from build123d import *

# Parameters (mm, degrees)
BOSS_EXTRUDE1_DEPTH             = 33.909
CUT_EXTRUDE1_DEPTH              = 70.971972376
BOSS_EXTRUDE2_REACH             = 67.168
BOSS_EXTRUDE2_DIRECTION_2_REACH = 67.168
SKETCH3_R                       = 2.25
CUT_EXTRUDE2_DEPTH              = 62.483683724
SKETCH5_R                       = 4.125
CUT_EXTRUDE3_DEPTH              = 62.483683724
BOSS_EXTRUDE3_DEPTH             = 3.175
CHAMFER1_SIZE                   = 3.175
CUT_EXTRUDE4_DEPTH              = 81.960563335
CUT_EXTRUDE5_DEPTH              = 66.16805579
CUT_EXTRUDE5_DEPTH_BACK         = 66.16805579
SKETCH8_R                       = 2.54
SKETCH8_R_2                     = 1.7
SKETCH8_3_R                     = 11.0998
SKETCH8_3_R_2                   = 2.54
CUT_EXTRUDE6_DEPTH              = 2.286
CUT_EXTRUDE7_DEPTH              = 81.960563335
CUT_EXTRUDE7_DEPTH_BACK         = 81.960563335
SKETCH9_R                       = 4.445
SKETCH10_W                      = 15.875
SKETCH10_H                      = 11.092
BOSS_EXTRUDE4_DEPTH             = 8
CUT_EXTRUDE8_DEPTH              = 8
SKETCH12_W                      = 12.7
SKETCH12_H                      = 7.917
CUT_EXTRUDE9_DEPTH              = 18.286
CUT_EXTRUDE10_DEPTH             = 8
FILLET1_R                       = 0.79375
CUT_EXTRUDE11_REACH             = 71.954
CUT_EXTRUDE11_END_RADIUS        = 8.60425
SKETCH15_R                      = 1.5
CUT_EXTRUDE12_REACH             = 68.541
BOSS_EXTRUDE6_REACH             = 76.111


# Read off the part's stored shape, not the designer's step: Mirror1
with BuildPart() as part:
    # Sketch1 → Boss-Extrude1 (new, symmetric)
    with BuildSketch(Plane(origin=(0, 0, 0), x_dir=(0, 0, -1), z_dir=(1, 0, 0))):
        Polygon((0, -21.4015), (0, 19.8735), (4.7625, 19.8735), (4.7625, 11.8735), (51.3715, 11.8735), (51.3715, 0), (4.7625, 0), (4.7625, -21.4015), align=None)
    extrude(amount=BOSS_EXTRUDE1_DEPTH, both=True)

    # Sketch2 → Cut-Extrude1 (cut, symmetric)
    with BuildSketch(Plane(origin=(0, 11.8735, 0), x_dir=(1, 0, 0), z_dir=(0, 1, 0))):
        Polygon((33.909, 4.7625), (29.6545, 4.7625), (24.892, 9.525), (24.892, 42.644487102), (16.164987102, 51.3715), (23.7109, 51.3715), (33.909, 51.3715), align=None)
    extrude(amount=CUT_EXTRUDE1_DEPTH, both=True, mode=Mode.SUBTRACT)

    # Boss-Extrude2: up to this face of the body (flat: up to its plane)
    boss_extrude2_end = Plane(part.part.faces().sort_by_distance((0, -21.4015, -2.38125))[0])
    # Sketch4 → Boss-Extrude2 (add, up to the picked face)
    with BuildSketch(Plane.XZ, mode=Mode.PRIVATE) as boss_extrude2_sk1:
        Polygon((24.892, -9.525), (29.6545, -4.7625), (24.892, -4.7625), align=None)
    boss_extrude2_tool1 = split(extrude(boss_extrude2_sk1.sketch, amount=BOSS_EXTRUDE2_REACH, mode=Mode.PRIVATE), bisect_by=boss_extrude2_end, keep=Keep.BOTH, mode=Mode.PRIVATE)
    add(boss_extrude2_tool1.solids().sort_by(Axis((26.4795, 0, -6.35), (0, -1, 0)))[0])

    # Boss-Extrude2 direction 2: up to this face of the body (flat: up to its plane)
    boss_extrude2_direction_2_end = Plane(part.part.faces().sort_by_distance((0, 19.8735, -2.38125))[0])
    # Sketch4 → Boss-Extrude2 direction 2 (add, up to the picked face)
    with BuildSketch(Plane.XZ, mode=Mode.PRIVATE) as boss_extrude2_direction_2_sk1:
        Polygon((24.892, -9.525), (29.6545, -4.7625), (24.892, -4.7625), align=None)
    boss_extrude2_direction_2_tool1 = split(extrude(boss_extrude2_direction_2_sk1.sketch, amount=-BOSS_EXTRUDE2_DIRECTION_2_REACH, mode=Mode.PRIVATE), bisect_by=boss_extrude2_direction_2_end, keep=Keep.BOTH, mode=Mode.PRIVATE)
    add(boss_extrude2_direction_2_tool1.solids().sort_by(Axis((26.4795, 0, -6.35), (0, 1, 0)))[0])

    # Sketch3 → Cut-Extrude2 (cut, symmetric)
    with BuildSketch(Plane(origin=(0, 0, -4.7625), x_dir=(-1, 0, 0), z_dir=(0, 0, -1))):
        with Locations(Location((-29.4005, 10.3485, 0), (0, 0, 90))):
            Circle(SKETCH3_R)
        with Locations(Location((-29.4005, -11.8765, 0), (0, 0, 90))):
            Circle(SKETCH3_R)
        Polygon((-29.6545, 19.8735), (-33.909, 15.619), (-33.909, 19.8735), align=None)
        Polygon((-33.909, 5.078), (-29.6545, 0.8235), (-29.6545, -2.3515), (-33.909, -6.606), align=None)
        Polygon((-33.909, -17.147), (-29.6545, -21.4015), (-33.909, -21.4015), align=None)
    extrude(amount=CUT_EXTRUDE2_DEPTH, both=True, mode=Mode.SUBTRACT)

    # Sketch5 → Cut-Extrude3 (cut, through all)
    with BuildSketch(Plane(origin=(0, 0, -4.7625), x_dir=(-1, 0, 0), z_dir=(0, 0, -1))):
        with Locations((-29.4005, 10.3485)):
            Circle(SKETCH5_R)
        with Locations((-29.4005, -11.8765)):
            Circle(SKETCH5_R)
    extrude(amount=CUT_EXTRUDE3_DEPTH, mode=Mode.SUBTRACT)

    # Sketch6 → Boss-Extrude3 (add)
    with BuildSketch(Plane.ZY.offset(-24.892)):
        Polygon((-4.7625, -21.4015), (-4.7625, 0), (-42.644487102, 0), align=None)
    extrude(amount=BOSS_EXTRUDE3_DEPTH)

    # Chamfer1
    chamfer1_edges = [part.edges().sort_by_distance(p)[0] for p in [
        (21.717, -10.70075, -4.7625),
    ]]
    chamfer(chamfer1_edges, length=CHAMFER1_SIZE)

    # Sketch7 → Cut-Extrude4 (cut, symmetric)
    with BuildSketch(Plane(origin=(24.892, 0, 0), x_dir=(0, 0, -1), z_dir=(1, 0, 0))):
        Polygon((9.525, -18.71091665), (4.7625, -21.4015), (9.525, -21.4015), align=None)
    extrude(amount=CUT_EXTRUDE4_DEPTH, both=True, mode=Mode.SUBTRACT)

    # Mirror1
    split(bisect_by=Plane(origin=(0, 0, 0), x_dir=(0, 0, 1), z_dir=(1, 0, 0)), keep=Keep.TOP)

    # Mirror1 2: part across plane


with BuildPart() as part_1:
    add(part.part)
    add(part.part.mirror(Plane(origin=(0, 0, 0), x_dir=(0, 0, 1), z_dir=(1, 0, 0))))

    # Sketch8 → Cut-Extrude5 (cut, two sides: drawn at the far end of the back side and taken through both)
    with BuildSketch(Plane.XZ.offset(-CUT_EXTRUDE5_DEPTH_BACK)):
        with Locations(Location((0, -26.4795, 0), (0, 0, 270))):
            Circle(SKETCH8_R)
        with Locations(Location((15.5, -10.9795, 0), (0, 0, 270))):
            Circle(SKETCH8_R_2)
        with Locations(Location((15.5, -41.9795, 0), (0, 0, 270))):
            Circle(SKETCH8_R_2)
        with Locations(Location((-15.5, -41.9795, 0), (0, 0, 270))):
            Circle(SKETCH8_R_2)
        with Locations(Location((-15.5, -10.9795, 0), (0, 0, 270))):
            Circle(SKETCH8_R_2)
    extrude(amount=CUT_EXTRUDE5_DEPTH + CUT_EXTRUDE5_DEPTH_BACK, mode=Mode.SUBTRACT)

    # Sketch8<3> → Cut-Extrude6 (cut)
    with BuildSketch(Plane.XZ):
        with Locations(Location((0, -26.4795, 0), (0, 0, 270))):
            Circle(SKETCH8_3_R)
        with Locations(Location((0, -26.4795, 0), (0, 0, 270))):
            Circle(SKETCH8_3_R_2, mode=Mode.SUBTRACT)
    extrude(amount=-CUT_EXTRUDE6_DEPTH, mode=Mode.SUBTRACT)

    # Sketch9 → Cut-Extrude7 (cut, two sides: drawn at the far end of the back side and taken through both)
    with BuildSketch(Plane(origin=(24.892, 0, 0), x_dir=(0, 0, -1), z_dir=(1, 0, 0)).offset(-CUT_EXTRUDE7_DEPTH_BACK)):
        with Locations((35.8345, 11.8735)):
            Circle(SKETCH9_R)
    extrude(amount=CUT_EXTRUDE7_DEPTH + CUT_EXTRUDE7_DEPTH_BACK, mode=Mode.SUBTRACT)

    # Sketch10 → Boss-Extrude4 (add)
    with BuildSketch(Plane(origin=(0, 11.8735, 0), x_dir=(1, 0, 0), z_dir=(0, 1, 0))):
        with Locations((0, 45.8255)):
            Rectangle(SKETCH10_W, SKETCH10_H)
    extrude(amount=BOSS_EXTRUDE4_DEPTH)

    # Sketch11 → Cut-Extrude8 (cut)
    with BuildSketch(Plane(origin=(0, 11.8735, 0), x_dir=(1, 0, 0), z_dir=(0, 1, 0))):
        with BuildLine():
            Line((-7.9375, 40.2795), (7.9375, 40.2795))
            Line((7.9375, 40.2795), (11.26, 31.3895))
            Line((11.26, 31.3895), (11.26, 23.880766055))
            Line((11.26, 23.880766055), (2.086105319, 20.616574655))
            ThreePointArc((2.086105319, 20.616574655), (1.0584764, 20.347179337), (0, 20.2565))
            Line((0, 20.2565), (0, 17.87525))
            ThreePointArc((0, 17.87525), (-6.847467237, 21.26938383), (-8.292669268, 28.774005279))
            ThreePointArc((-8.292669268, 28.774005279), (-8.02669792, 30.069750228), (-7.9375, 31.3895))
            Line((-7.9375, 31.3895), (-7.9375, 40.2795))
        make_face()
    extrude(amount=-CUT_EXTRUDE8_DEPTH, mode=Mode.SUBTRACT)

    # Sketch12 → Cut-Extrude9 (cut)
    with BuildSketch(Plane.XZ):
        with Locations((0, -45.8255)):
            Rectangle(SKETCH12_W, SKETCH12_H)
    extrude(amount=-CUT_EXTRUDE9_DEPTH, mode=Mode.SUBTRACT)

    # Sketch13 → Cut-Extrude10 (cut)
    with BuildSketch(Plane(origin=(0, 11.8735, 0), x_dir=(1, 0, 0), z_dir=(0, 1, 0))):
        with BuildLine():
            Line((14.308, 21.730089687), (3.048, 17.723634801))
            Line((3.048, 17.723634801), (3.048, 15.232961596))
            ThreePointArc((3.048, 15.232961596), (-7.751371841, 17.779433066), (-11.522356749, 28.2145))
            Line((-11.522356749, 28.2145), (-21.717, 28.2145))
            Line((-21.717, 28.2145), (-21.717, 9.525))
            Line((-21.717, 9.525), (-21.717, 7.9375))
            Line((-21.717, 7.9375), (-20.152961933, 7.9375))
            ThreePointArc((-20.152961933, 7.9375), (-18.873886587, 8.584722111), (-18.637766637, 9.998644872))
            ThreePointArc((-18.637766637, 9.998644872), (-15.996109076, 14.229351079), (-12.2125, 10.9795))
            ThreePointArc((-12.2125, 10.9795), (-12.250148921, 10.483390924), (-12.362233363, 9.998644872))
            ThreePointArc((-12.362233363, 9.998644872), (-12.126113413, 8.584722111), (-10.847038067, 7.9375))
            Line((-10.847038067, 7.9375), (10.847038067, 7.9375))
            ThreePointArc((10.847038067, 7.9375), (12.126113413, 8.584722111), (12.362233363, 9.998644872))
            ThreePointArc((12.362233363, 9.998644872), (15.003890924, 14.229351079), (18.7875, 10.9795))
            ThreePointArc((18.7875, 10.9795), (18.749851079, 10.483390924), (18.637766637, 9.998644872))
            ThreePointArc((18.637766637, 9.998644872), (18.873886587, 8.584722111), (20.152961933, 7.9375))
            Line((20.152961933, 7.9375), (21.717, 7.9375))
            Line((21.717, 7.9375), (21.717, 9.525))
            Line((21.717, 9.525), (21.717, 28.2145))
            Line((21.717, 28.2145), (14.308, 28.2145))
            Line((14.308, 28.2145), (14.308, 21.730089687))
        make_face()
    extrude(amount=-CUT_EXTRUDE10_DEPTH, mode=Mode.SUBTRACT)

    # Fillet1
    fillet1_edges = [part_1.edges().sort_by_distance(p)[0] for p in [
        (3.048, 3.8735, -16.478298199),
        (8.678, 3.8735, -19.726862244),
        (14.308, 3.8735, -24.972294843),
        (12.126113413, 3.8735, -8.584722111),
        (-18.873886587, 3.8735, -8.584722111),
        (-16.619678375, 3.8735, -28.2145),
        (-7.751371841, 3.8735, -17.779433066),
        (18.0125, 3.8735, -28.2145),
        (21.717, 3.8735, -18.076),
        (20.934980967, 3.8735, -7.9375),
        (18.873886587, 3.8735, -8.584722111),
        (15.003890924, 3.8735, -14.229351079),
        (0, 3.8735, -7.9375),
        (-12.126113413, 3.8735, -8.584722111),
        (-15.996109076, 3.8735, -14.229351079),
        (-20.934980967, 3.8735, -7.9375),
        (-21.717, 3.8735, -18.076),
    ]]
    fillet(fillet1_edges, radius=FILLET1_R - 0.0001)  # a hair under: the kernel refuses the full size

    # Cut-Extrude11: up to this cylinder (the profile starts outside it)
    cut_extrude11_end = Plane(origin=(0, 11.8735, -26.4795), z_dir=(0, 1, 0)) * Cylinder(CUT_EXTRUDE11_END_RADIUS, 162.1165, mode=Mode.PRIVATE)
    # Sketch15 → Cut-Extrude11 (cut, up to the surface)
    with BuildSketch(Plane(origin=(-6.946964947, 0, 1.224937354), x_dir=(0, 1, 0), z_dir=(-0.9848077530122085, 0, 0.17364817766692803)), mode=Mode.PRIVATE) as cut_extrude11_sk1:
        with Locations((11.8735, 26.077216896)):
            Circle(SKETCH15_R)
    cut_extrude11_tool1 = extrude(cut_extrude11_sk1.sketch, amount=-CUT_EXTRUDE11_REACH, mode=Mode.PRIVATE) - cut_extrude11_end
    add(cut_extrude11_tool1.solids().sort_by_distance((-11.475226, 11.8735, -24.456108))[0], mode=Mode.SUBTRACT)

    # Sketch16 → Cut-Extrude12 (cut, up to next)
    with BuildSketch(Plane(origin=(0, 3.8735, 0), x_dir=(1, 0, 0), z_dir=(0, 1, 0)), mode=Mode.PRIVATE) as cut_extrude12_sk1:
        with BuildLine():
            ThreePointArc((8.62682, 26.4795), (6.100082922, 32.579582922), (0, 35.10632))
            ThreePointArc((0, 35.10632), (-1.05, 34.05632), (0, 33.00632))
            ThreePointArc((0, 33.00632), (4.615158682, 31.094658682), (6.52682, 26.4795))
            ThreePointArc((6.52682, 26.4795), (7.57682, 25.4295), (8.62682, 26.4795))
        make_face()
    cut_extrude12_tool1 = extrude(cut_extrude12_sk1.sketch, amount=-CUT_EXTRUDE12_REACH, mode=Mode.PRIVATE) & part_1.part
    add(cut_extrude12_tool1.solids().sort_by_distance((4.697563, 3.8735, -31.177063))[0], mode=Mode.SUBTRACT)

    # Sketch17 → Boss-Extrude6 (add, up to next)
    with BuildSketch(Plane(origin=(0, 19.8735, 0), x_dir=(1, 0, 0), z_dir=(0, 1, 0)), mode=Mode.PRIVATE) as boss_extrude6_sk1:
        with BuildLine():
            Line((-6.35, 40.2795), (6.35, 40.2795))
            ThreePointArc((6.35, 40.2795), (5.487477355, 40.103743072), (4.7625, 39.6045))
            ThreePointArc((4.7625, 39.6045), (4.037522645, 39.105256928), (3.175, 38.9295))
            Line((3.175, 38.9295), (-3.175, 38.9295))
            ThreePointArc((-3.175, 38.9295), (-4.037522645, 39.105256928), (-4.7625, 39.6045))
            ThreePointArc((-4.7625, 39.6045), (-5.487477355, 40.103743072), (-6.35, 40.2795))
        make_face()
    boss_extrude6_tool1 = extrude(boss_extrude6_sk1.sketch, amount=-BOSS_EXTRUDE6_REACH, mode=Mode.PRIVATE) - part_1.part
    add(boss_extrude6_tool1.solids().sort_by_distance((0, 19.8735, -39.653988))[0])


solid = part_1.part
Can you work these out from the model? Positions are in its coordinate system, mm. A direction names the side the tool comes from. Give positions to 0.01 mm unless a question says otherwise; leave off trailing zeros. Loops run counter-clockwise (first coordinate to the right, second up) from the corner with the lowest first, then second, coordinate; pieces in that order, holes last. Notation, with made-up numbers: M -10.5,69.5 L 48.5,69.5 A21 ccw 48.5,106.5 Z; hole C 22.5,-25 d3. An arc over 180 degrees is marked long. One line per item, written item: value. Start each with the question number.
1) If we section it at A-A, the plane z = -47.5: Write out the boundary of the cut face in (x, y).
2) If we section it at B-B, the plane x = -23: Write out the boundary of the cut face in (y, z) (1 decimal), and give its area (3 significant figures).
3) If I drill on line 1 (X direction, y = -9, z = -21); line 2 (Z direction, x = 15, y = 2); line 3 (Z direction, x = 15.5, y = 8.5), over which ranges is the centre line in solid material (lowest first)? Write a range as [from, to].
4) On a 3-axis mill with a long thin cutter (end or side, diameter ignored), from which of +Z, -Z, +X, -X, +Y, -Y can I reach the whole of each face in a straight line? I mean faces 1 (the face through (14, 11.874, -46)), 2 (the face through (-2, 2.286, -24)), 3 (the face through (-31.81, 2.98, -2.35)), 4 (the face through (0, 8, -7.938)), 5 (the face through (-24.892, 16, -7)). Say none if no direction works.
5) I'm going to push flat-ended pins straight in: pin 1 (2 mm diameter, centred on y = 0.5, z = -26.5, fed in from -X); pin 2 (15.5 mm diameter, centred on y = -8, z = -20, fed in from +X); pin 3 (2 mm diameter, centred on x = -10.5, y = -3, fed in from +Z); pin 4 (1 mm diameter, centred on x = 0.5, z = -13.5, fed in from -Y). Where does each tip first touch, or does it pass through?
6) Thinking about a two-plate mould opening in Z: for faces 6 (the face through (-26.711, -0.475, -7.706)), 7 (the face through (-24.892, 0, -23)), 8 (the face through (0, 8, -19)), which applies, +Z half, -Z half, draft (parallel to the pull), parting line (faces both ways), or undercut?
Completed:
1. outline: M -20.04,0 L -6.35,0 L -6.35,18.29 L 6.35,18.29 L 6.35,0 L 20.04,0 L 20.04,11.87 L 7.94,11.87 L 7.94,19.87 L -7.94,19.87 L -7.94,11.87 L -20.04,11.87 Z
2. outline: M -21.4,-4.8 L 0,-42.6 L 0,-44.5 L 11.9,-44.5 L 11.9,-40.3 A4.4 cw 11.9,-31.4 L 11.9,-4.8 L 19.9,-4.8 L 19.9,0 L -21.4,0 Z
2. area: 1,040 mm^2
3. line 1: x = [-24.89, -21.72], [21.72, 24.89]
3. line 2: z = [-51.37, -43.6], [-40.35, -12.6], [-9.35, 0]
3. line 3: z = [-51.37, -43.68], [-40.28, -38.73], [-32.94, -28.21], [-14.27, -12.68], [-9.28, 0]
4. face 1: -Z, +X, +Y
4. face 2: -Y
4. face 3: +Z, -Z, -X
4. face 4: +Y
4. face 5: -Z, +Y
5. pin 1: stops at x = -24.89
5. pin 2: stops at x = 24.89
5. pin 3: stops at z = 0
5. pin 4: stops at y = 0
6. face 6: -Z half
6. face 7: draft
6. face 8: undercut
